Geometry: see drawing. Coordinates: mm, zero at the bounding-box minimum. A direction names the side the tool comes from. Round coordinates to 2 decimals unless told otherwise and drop trailing zeros. Loops run counter-clockwise (first coordinate to the right, second up) from the corner with the lowest first, then second, coordinate; pieces in that order, holes last. Notation, with made-up numbers: (85.5, 17.25) -> (106.5, 17.25) arc R28 cw to (106.5, 54.25) -> close; hole circle Ø4 at (-3, -32). An arc over 180 degrees is marked (long way). Write item = value, one per line.
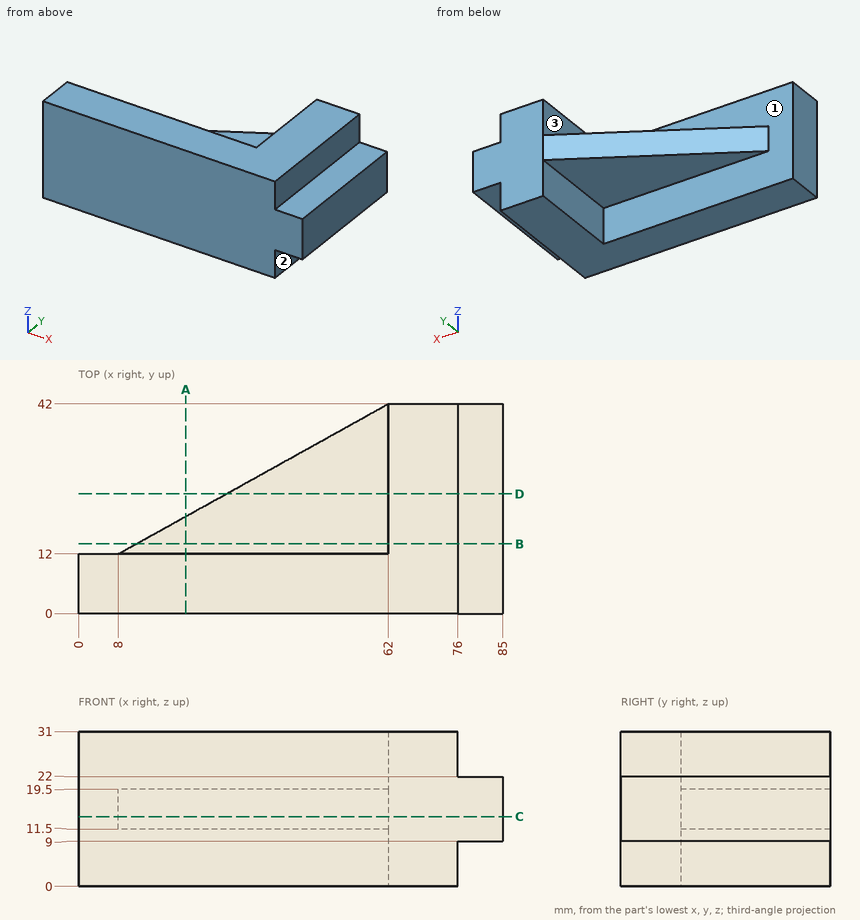
1. Section query C-C (z = 14). Return the cut outline in (x, y).
Evaluation:
outline = (0, 0) -> (85, 0) -> (85, 42) -> (62, 42) -> (8, 12) -> (0, 12) -> close
2. Section query A-A (x = 21.5). Return the cut outline in (y, z), then the cut area to 3 significant figures.
Evaluation:
outline = (0, 0) -> (12, 0) -> (12, 11.5) -> (19.5, 11.5) -> (19.5, 19.5) -> (12, 19.5) -> (12, 31) -> (0, 31) -> close
area = 432 mm²
3. Section query B-B (y = 14). Return the cut outline in (x, z), then the cut area to 3 significant figures.
Evaluation:
outline = (11.6, 11.5) -> (62, 11.5) -> (62, 0) -> (76, 0) -> (76, 9) -> (85, 9) -> (85, 22) -> (76, 22) -> (76, 31) -> (62, 31) -> (62, 19.5) -> (11.6, 19.5) -> close
area = 954 mm²
4. Set-up query: the marked faces 1, 2 and 3. Return all of +Z, -Z, +X, -X, +Y, -Y with unobstructed straight access to the full face (end or side cutting, diameter ignored); none if empty.
Evaluation:
face_1 = -X, +Y
face_2 = -Z, +X, +Y, -Y
face_3 = +Z, -X, +Y
5. Contact query for flat-ended pins moving along their axis: pin 1 Ø9.5 at (x, z) = (16, 21.5) entering from +Y; pin 2 Ø10 at (y, z) = (35, 3) entering from -X; pin 3 Ø8 at (x, z) = (40.5, 13.5) entering from +Y; pin 4 Ø6 at (x, y) = (59.5, 29) entering from -Z. Output: stop coordinate, or through.
Evaluation:
pin_1 = 18.84
pin_2 = 62
pin_3 = 32.28
pin_4 = 0
6. Section query D-D (y = 24). Return the cut outline in (x, z), then the cut area to 3 significant figures.
Evaluation:
outline = (29.6, 11.5) -> (62, 11.5) -> (62, 0) -> (76, 0) -> (76, 9) -> (85, 9) -> (85, 22) -> (76, 22) -> (76, 31) -> (62, 31) -> (62, 19.5) -> (29.6, 19.5) -> close
area = 810 mm²
7. Line query: probe 1 along Z at (x, y) = (79, 34.5); probe 2 along Y at (x, z) = (17.5, 8); probe 3 along Z at (x, y) = (54, 21). Output: solid intervals per line, ascending. Write a range as from..to.
Evaluation:
probe_1 = 9..22
probe_2 = 0..12
probe_3 = 11.5..19.5
